from build123d import *

# Parameters (mm, degrees)
SKETCH1_R           = 92.5
BOSS_EXTRUDE1_DEPTH = 16
SKETCH2_R           = 27.5
CUT_EXTRUDE1_DEPTH  = 132.789605053
SKETCH3_R           = 6.047272506
CUT_EXTRUDE2_DEPTH  = 14.926051
CIRPATTERN1_START   = 1.073948621
CIRPATTERN1_DEPTH   = 14.926051379


# Read off the part's stored shape, not the designer's step: CirPattern1
with BuildPart() as part:
    # Sketch1 → Boss-Extrude1 (new body)
    with BuildSketch(Plane(origin=(0, 0, 0), x_dir=(1, 0, 0), z_dir=(0, 1, 0))):
        with Locations(Location((0, 0, 0), (0, 0, 270))):
            Circle(SKETCH1_R)
    extrude(amount=BOSS_EXTRUDE1_DEPTH)

    # Sketch2 → Cut-Extrude1 (cut, through all)
    with BuildSketch(Plane(origin=(0, 0, 0), x_dir=(1, 0, 0), z_dir=(0, 1, 0))):
        with Locations(Location((0, 0, 0), (0, 0, 270))):
            Circle(SKETCH2_R)
    extrude(amount=CUT_EXTRUDE1_DEPTH, mode=Mode.SUBTRACT)

    # Sketch3 → Cut-Extrude2 (cut)
    with BuildSketch(Plane(origin=(0, 16, 0), x_dir=(1, 0, 0), z_dir=(0, 1, 0))):
        with Locations((-32.634958459, 0)):
            Circle(SKETCH3_R)
    extrude(amount=-CUT_EXTRUDE2_DEPTH, mode=Mode.SUBTRACT)

    # CirPattern1 outline → CirPattern1 (cut)
    with BuildSketch(Plane(origin=(0, 0, 0), x_dir=(1, 0, 0), z_dir=(0, 1, 0)).offset(CIRPATTERN1_START)):
        with BuildLine():
            ThreePointArc((11.136289906, 25.144244811), (13.75, 23.815698604), (16.207409813, 22.216432368))
            ThreePointArc((16.207409813, 22.216432368), (19.341115482, 33.49979469), (11.136289906, 25.144244811))
        make_face()
        with BuildLine():
            ThreePointArc((16.207409813, -22.216432368), (13.75, -23.815698604), (11.136289906, -25.144244811))
            ThreePointArc((11.136289906, -25.144244811), (19.341115482, -33.49979469), (16.207409813, -22.216432368))
        make_face()
    extrude(amount=CIRPATTERN1_DEPTH, mode=Mode.SUBTRACT)


solid = part.part
CAD build for the part. Positions are in the model's coordinates, mm. A direction names the side the tool comes from. Give positions to 0.01 mm unless a question says otherwise; leave off trailing zeros. Write each loop counter-clockwise with the first axis right and the second up, starting at its lowest first coordinate (ties: lowest second). Pieces come first, ordered by that corner, then holes. Notation, with made-up numbers: (12.5, -31) - (60.5, -31) arc R13 ccw to (60.5, -6) - close; hole circle Ø1 at (86.5, -14). An arc over 180 degrees is marked (long way). Put each result on its own line as item: value.
(1) Saw through at C-C (x = -30). List the corners of the cut face in (y, z), then the cut area to 3 significant figures.
Working result:
outline: (0, -87.5) - (16, -87.5) - (16, -5.44) - (1.07, -5.44) - (1.07, 5.44) - (16, 5.44) - (16, 87.5) - (0, 87.5) - close
area: 2,640 mm^2
(2) Drop flat-ended pins along their axis: pin 1 Ø1.5 at (x, y) = (-55.5, 11.5) entering from -Z; pin 2 Ø8 at (y, z) = (2.5, -25.5) entering from +X; pin 3 Ø6 at (x, z) = (18.5, -29.5) entering from +Y. Give the stop position or say it passes through.
Working result:
pin 1: z = -74.56
pin 2: x = 89.97
pin 3: y = 1.07
(3) Saw through at B-B (x = -10). List the corners of the cut face in (y, z), then the cut area to 3 significant figures.
Working result:
outline: (0, -91.96) - (16, -91.96) - (16, -25.62) - (0, -25.62) - close; (0, 25.62) - (16, 25.62) - (16, 91.96) - (0, 91.96) - close
area: 2,120 mm^2
(4) Saw through at A-A (z = 0). List the corners of the cut face in (x, y).
Working result:
outline: (-92.5, 0) - (-27.5, 0) - (-27.5, 1.07) - (-38.68, 1.07) - (-38.68, 16) - (-92.5, 16) - close; (27.5, 0) - (92.5, 0) - (92.5, 16) - (27.5, 16) - close
(5) Saw through at D-D (z = -19.5). List the corners of the cut face in (x, y), then the cut area to 3 significant figures.
Working result:
outline: (-90.42, 0) - (-19.39, 0) - (-19.39, 16) - (-90.42, 16) - close; (19.39, 0) - (90.42, 0) - (90.42, 16) - (19.39, 16) - close
area: 2,270 mm^2
(6) Pull direction X, two halves, no side cores. Call faces 3 (the flat face through (22, 16, 19)), 4 (the cylindrical face through (-90.3, 7.89, -20.05)), 5 (the cylindrical face through (-38.68, 8.64, -0.22)), 6 (the cylindrical face through (-24.397, 7.888, 12.69)): released by +X, released by -X, zero draft, split by the parting line, or undercut.
Working result:
face 3: zero draft
face 4: split by the parting line
face 5: undercut
face 6: undercut
(7) Wall check: L1, parallel to X at y = 10, z = 22; L2, parallel to X at y = 3, z = 13; L3, parallel to Z at x = 8.5, y = 0.75. Give the ranges that are in metal, low to high.
Working result:
L1: -89.85 to -16.5, 16.5 to 89.85
L2: -91.58 to -24.23, 24.23 to 91.58
L3: -92.11 to -26.15, 26.15 to 92.11
(8) Tool access for faces 1 (the cylindrical face through (19.532, 8.432, -33.385)), 2 (the flat face through (22, 0, 19)): list every direction of +Z, -Z, +X, -X, +Y, -Y with a clear straight run to the whole face (end or side of a thin tool).
Working result:
face 1: +Y
face 2: +Z, -Z, +X, -X, -Y
